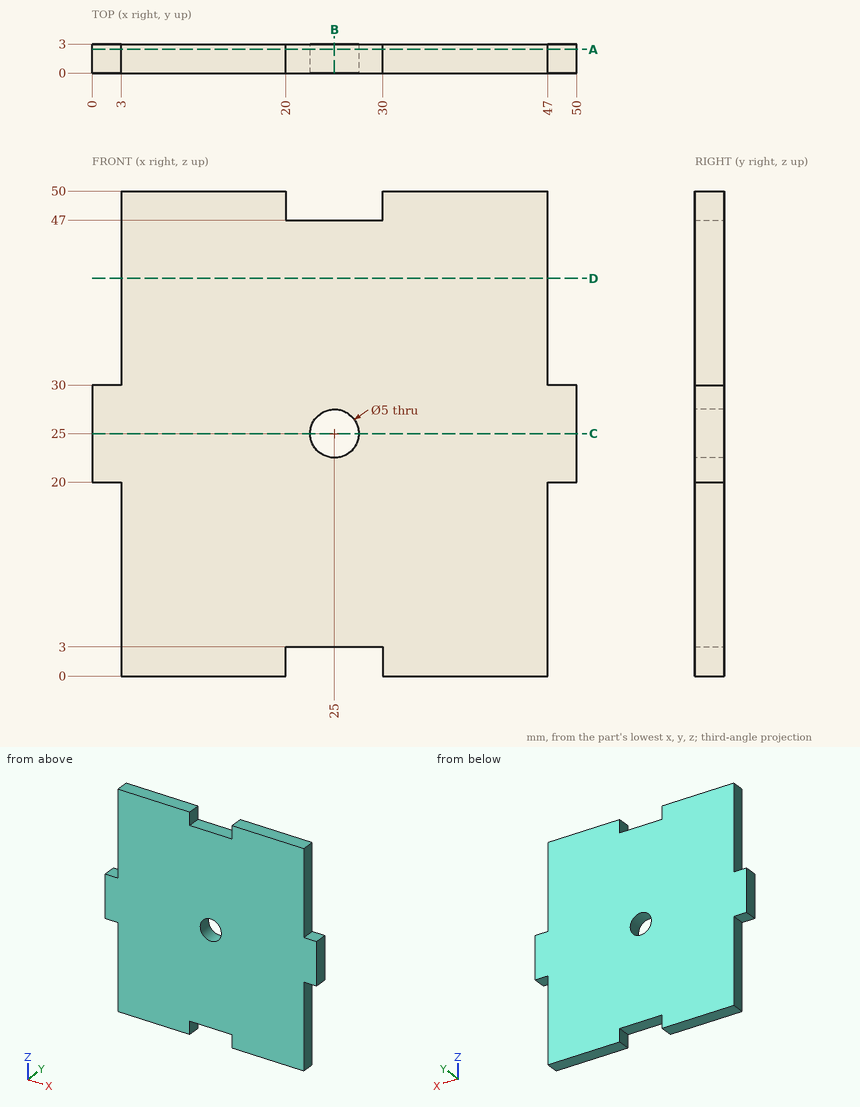
Geometry: see drawing. Coordinates: mm, zero at the bounding-box minimum. Coordinates: 2 decimals unless noted, no trailing zeros. Loops run counter-clockwise (first coordinate to the right, second up) from the corner with the lowest first, then second, coordinate; pieces in that order, holes last. Notation, with made-up numbers: (83, 61.25) - (89, 61.25) arc R28 cw to (89, 85.25) - close; hole circle Ø11 at (7.25, 24.5). An arc over 180 degrees is marked (long way). Answer as CSV lines item,"result".
1. Section C-C (z = 25). Return loops of the section in (x, y), then the cut area to 3 significant figures.
Established:
outline,"(0, 0) - (22.5, 0) - (22.5, 3) - (0, 3) - close; (27.5, 0) - (50, 0) - (50, 3) - (27.5, 3) - close"
area,"135 mm2"
2. Section D-D (z = 41). Return loops of the section in (x, y).
Established:
outline,"(3, 0) - (47, 0) - (47, 3) - (3, 3) - close"
3. Ray query, line 1 (Z direction, x = 25, y = 0.8); line 2 (X direction, y = 1.3, z = 36.5). Return the intervals inside material, ascending.
Established:
line 1,"z = 3 to 22.5, 27.5 to 47"
line 2,"x = 3 to 47"
4. Section B-B (x = 25). Return loops of the section in (y, z).
Established:
outline,"(0, 3) - (3, 3) - (3, 22.5) - (0, 22.5) - close; (0, 27.5) - (3, 27.5) - (3, 47) - (0, 47) - close"
5. Section A-A (y = 2.45). Return loops of the section in (x, z).
Established:
outline,"(0, 20) - (3, 20) - (3, 0) - (20, 0) - (20, 3) - (30, 3) - (30, 0) - (47, 0) - (47, 20) - (50, 20) - (50, 30) - (47, 30) - (47, 50) - (30, 50) - (30, 47) - (20, 47) - (20, 50) - (3, 50) - (3, 30) - (0, 30) - close; hole circle Ø5 at (25, 25)"
6. Contact query for flat-ended pins moving along their axis: pin 1 (4 mm diameter, centred on x = 25, z = 25, fed in from -Y); pin 2 (0.9 mm diameter, centred on x = 1, y = 1.5, fed in from -Z); pin 3 (0.9 mm diameter, centred on x = 1, y = 1.5, fed in from +Z); pin 4 (1.5 mm diameter, centred on y = 2, z = 7, fed in from +X). Output: stop coordinate, or through.
Established:
pin 1,"passes through"
pin 2,"stops at z = 20"
pin 3,"stops at z = 30"
pin 4,"stops at x = 47"
